from build123d import *

# Parameters (mm, degrees)
SKETCH_1_W              = 140
SKETCH_1_H              = 130
EXTRUDE_1_DEPTH         = 68
SKETCH_2_R              = 50
CUT_EXTRUDE_2_DEPTH     = 131
SKETCH_3_R              = 6.5
CUT_EXTRUDE_3_DEPTH     = 35
SKETCH_4_R              = 4
CUT_EXTRUDE_4_DEPTH     = 34
HOLE_WIZARD_M6_10_D     = 5
HOLE_WIZARD_M6_10_DEPTH = 15
HOLE_WIZARD_M6_10_TIP   = 1.502151548


with BuildPart() as part:
    # 草图1 → 凸台-拉伸1 (new body)
    with BuildSketch(Plane.XY):
        with Locations((70, -65)):
            Rectangle(SKETCH_1_W, SKETCH_1_H)
    extrude(amount=EXTRUDE_1_DEPTH)

    # 草图2 → 切除-拉伸2 (cut, through all)
    with BuildSketch(Plane(origin=(0, 0, 0), x_dir=(1, 0, 0), z_dir=(0, 1, 0))):
        with Locations((70, -65)):
            Circle(SKETCH_2_R)
    extrude(amount=-CUT_EXTRUDE_2_DEPTH, mode=Mode.SUBTRACT)

    # 草图3 → 切除-拉伸3 (cut)
    with BuildSketch(Plane.XY.offset(68)):
        with Locations((7.5, -28)):
            Circle(SKETCH_3_R)
        with Locations((132.5, -28)):
            Circle(SKETCH_3_R)
        with Locations((132.5, -68)):
            Circle(SKETCH_3_R)
        with Locations((132.5, -108)):
            Circle(SKETCH_3_R)
        with Locations((7.5, -68)):
            Circle(SKETCH_3_R)
        with Locations((7.5, -108)):
            Circle(SKETCH_3_R)
    extrude(amount=-CUT_EXTRUDE_3_DEPTH, mode=Mode.SUBTRACT)

    # 草图4 → 切除-拉伸4 (cut, through all)
    with BuildSketch(Plane.XY.offset(33)):
        with Locations((132.5, -28)):
            Circle(SKETCH_4_R)
        with Locations((7.5, -28)):
            Circle(SKETCH_4_R)
        with Locations((132.5, -68)):
            Circle(SKETCH_4_R)
        with Locations((132.5, -108)):
            Circle(SKETCH_4_R)
        with Locations((7.5, -68)):
            Circle(SKETCH_4_R)
        with Locations((7.5, -108)):
            Circle(SKETCH_4_R)
    extrude(amount=-CUT_EXTRUDE_4_DEPTH, mode=Mode.SUBTRACT)

    # M6 螺纹孔10
    with Locations(Plane.XY.offset(68)):
        with Locations((7.5, -11), (7.5, -47), (7.5, -83), (132.5, -83), (132.5, -47), (132.5, -11), (7.5, -119), (132.5, -119)):
            Hole(HOLE_WIZARD_M6_10_D / 2, depth=HOLE_WIZARD_M6_10_DEPTH)
            with Locations((0, 0, -(HOLE_WIZARD_M6_10_DEPTH + HOLE_WIZARD_M6_10_TIP / 2))):  # 118° drill point
                Cone(0, HOLE_WIZARD_M6_10_D / 2, HOLE_WIZARD_M6_10_TIP, mode=Mode.SUBTRACT)


solid = part.part
CAD build for the part. Positions are in the model's coordinates, mm. A direction names the side the tool comes from. Round coordinates to 2 decimals unless told otherwise and drop trailing zeros. Order: outer loops, then holes, each group sorted by start corner. A loop starts at its lowest first (then second) coordinate and runs counter-clockwise, first axis right, second up. Notation, with made-up numbers: M 30.5,-13.75 L 56.5,-13.75 A25 ccw 56.5,20.25 Z; hole C -8.5,-40 d8. An arc over 180 degrees is marked long. Use one line per item in the form item = value.
Q1. Saw through at A-A on y = -68. Give the cut face in (x, z).
Recorded:
outline = M 0,0 L 3.5,0 L 3.5,33 L 1,33 L 1,68 L 0,68 Z; M 11.5,0 L 128.5,0 L 128.5,33 L 126,33 L 126,68 L 119.91,68 A50 cw long 20.09,68 L 14,68 L 14,33 L 11.5,33 Z; M 136.5,0 L 140,0 L 140,68 L 139,68 L 139,33 L 136.5,33 Z
Q2. Saw through at D-D on z = 19. Give the cut face in (x, y).
Recorded:
outline = M 0,-130 L 50.4,-130 L 50.4,0 L 0,0 Z; M 89.6,-130 L 140,-130 L 140,0 L 89.6,0 Z; hole C 7.5,-108 d8; hole C 7.5,-68 d8; hole C 7.5,-28 d8; hole C 132.5,-108 d8; hole C 132.5,-68 d8; hole C 132.5,-28 d8
Q3. Probe L1, parallel to Y at x = 7, z = 10; L2, parallel to X at y = -123, z = 65; L3, parallel to X at y = -31.5, z = 35. List the from-to ranges inside material, lowest first.
Recorded:
L1 = -130 to -111.97, -104.03 to -71.97, -64.03 to -31.97, -24.03 to 0
L2 = 0 to 20, 120 to 140
L3 = 0 to 2.02, 12.98 to 30, 110 to 127.02, 137.98 to 140
Q4. Two-plate mould, pull along Y, no slides. Class faces 1 (the flat face through (69, -130, 11)), 2 (the flat face through (140, -66, 34)), 3 (the cylindrical face through (130.115, -118.249, 60.395)): +Y half, -Y half, draft (parallel to the pull), parting line (faces both ways), or undercut.
Recorded:
face_1 = -Y half
face_2 = draft
face_3 = undercut
Q5. Saw through at B-B on z = 49. Give the cut face in (x, y), then the cut area to 3 significant figures.
Recorded:
outline = M 0,-130 L 22.63,-130 L 22.63,0 L 0,0 Z; M 117.37,-130 L 140,-130 L 140,0 L 117.37,0 Z; hole C 7.5,-108 d13; hole C 7.5,-68 d13; hole C 7.5,-28 d13; hole C 132.5,-108 d13; hole C 132.5,-68 d13; hole C 132.5,-28 d13
area = 5,090 mm^2
Q6. Which spindle directions (+Z, -Z, +X, -X, +Y, -Y) get a long thin tool onto all of the face, cutting with end or side? Do faces 4 (the flat face through (69, 0, 11)), 5 (the cylindrical face through (126, -108, 51)). Say none if no direction does.
Recorded:
face_4 = +Z, -Z, +X, -X, +Y
face_5 = +Z
Q7. Flat gauge pins, fed straight in: P1, Ø6, axis at x = 7.5, y = -11, coming from the -Z side; P2, Ø5, axis at x = 7.5, y = -108, coming from the -Z side; P3, Ø9, axis at x = 132.5, y = -68, coming from the +Z side; P4, Ø10, axis at x = 96, y = -63, coming from the +Z side. Where does each tip first touch, or does it go through?
Recorded:
P1 = 0
P2 = through
P3 = 33
P4 = 25.77
Q8. Saw through at C-C on y = -99. Give the cut face in (x, z), then the cut area to 3 significant figures.
Recorded:
outline = M 0,0 L 140,0 L 140,68 L 119.91,68 A50 cw long 20.09,68 L 0,68 Z
area = 5,290 mm^2
